Autodesk Inventor part; units mm, degrees
ref_plane "Work Plane1" through (-19.4127, 25.0373, 33.395) normal (0, 0, -1) x (0, 1, 0)
ref_plane "YZ Plane" through (0, 0, 0) normal (1, 0, 0) x (0, 1, 0)
ref_plane "XZ Plane" through (0, 0, 0) normal (0, 1, 0) x (-1, 0, 0)
sketch "Sketch1" plane through (0, 0, 0) normal (0, 0, 1) x (1, 0, 0)
  line L0 (34.925, 95.25) -> (-34.925, 95.25)
  line L1 (-34.925, 95.25) -> (-34.925, 82.55)
  line L2 (-34.925, 82.55) -> (34.925, 82.55)
  line L3 (34.925, 82.55) -> (34.925, 95.25)
  circle A0 centre (-29.0032, 88.9) radius 2.3812
  circle A1 centre (29.0032, 88.9) radius 2.3812
  line L4 (34.925, 6.35) -> (-34.925, 6.35)
  line L5 (-34.925, 6.35) -> (-34.925, -6.35)
  line L6 (-34.925, -6.35) -> (34.925, -6.35)
  line L7 (34.925, -6.35) -> (34.925, 6.35)
  circle A2 centre (-29.0032, 0) radius 2.3812
  circle A3 centre (29.0032, 0) radius 2.3812
  line L8 (34.925, 82.55) -> (34.925, 6.35)
  line L9 (-34.925, 6.35) -> (-34.925, 82.55)
  circle A4 centre (0, 44.45) radius 22.225
  point P0 (0, 0)
  dimension "d0" = 44.45
extrude "Extrusion1" add sketch "Sketch1" along normal blind 12.7
ref_plane "Work Plane1" through (-19.4127, 25.0373, 33.395) normal (0, 0, -1) x (0, 1, 0)
properties part number "Encoder Mount Y"
Verification items for the finished model (mm, model axes). Coordinates: 2 decimals unless noted, no trailing zeros. Order: outer loops, then holes, each group sorted by start corner. A loop starts at its lowest first (then second) coordinate and runs counter-clockwise, first axis right, second up. Notation, with made-up numbers: M -14.5,78.5 L 1.5,78.5 A17 cw 1.5,91.5 Z; hole C -24.5,-25 d2. An arc over 180 degrees is marked long. Return JSON: item names as keys, results as strings.
1) Thickness scan on L1, parallel to Y at x = 0, z = 9.75 (3 decimals); L2, parallel to Y at x = -31, z = 7.75; L3, parallel to Y at x = 30, z = 4. Record the ranges inside material, lowest first. Write a range as [from, to].
Answer list:
{"L1": "[-6.35, 22.225], [66.675, 95.25]", "L2": "[-6.35, -1.3], [1.3, 87.6], [90.2, 95.25]", "L3": "[-6.35, -2.16], [2.16, 86.74], [91.06, 95.25]"}
2) Cross-section at D-D, the plane z = 5.5. Record the boundary of the cut face in (x, y) (3 decimals), and give its area (3 significant figures).
Answer list:
{"outline": "M -34.925,-6.35 L 34.925,-6.35 L 34.925,95.25 L -34.925,95.25 Z; hole C -29.003,0 d4.762; hole C -29.003,88.9 d4.762; hole C 0,44.45 d44.45; hole C 29.003,0 d4.762; hole C 29.003,88.9 d4.762", "area": "5,470 mm2"}
3) Gauge pin test, flat end, axial feed: pin 1 (5.5 mm diameter, centred on x = 29, y = 88.9, fed in from +Z). Record the tip position at first contact, or that the pin passes through.
Answer list:
{"pin 1": "z = 12.7"}
4) Release check for a two-part mould opening along X. For faces 1 (the flat face through (0, 95.25, 6)), 2 (the flat face through (34.925, 44, 6)), 3 (the flat face through (-34.925, 45, 6)), 4 (the cylindrical face through (-31.382, -0.105, 6.261)) record: +X half, -X half, draft (parallel to the pull), parting line (faces both ways), or undercut.
Answer list:
{"face 1": "draft", "face 2": "+X half", "face 3": "-X half", "face 4": "undercut"}
5) Cross-section at B-B, the plane x = 0. Record the boundary of the cut face in (y, z) (3 decimals).
Answer list:
{"outline": "M -6.35,0 L 22.225,0 L 22.225,12.7 L -6.35,12.7 Z; M 66.675,0 L 95.25,0 L 95.25,12.7 L 66.675,12.7 Z"}
6) Cross-section at C-C, the plane y = 88.9. Record the boundary of the cut face in (x, z) (3 decimals), and give its area (3 significant figures).
Answer list:
{"outline": "M -34.925,0 L -31.384,0 L -31.384,12.7 L -34.925,12.7 Z; M -26.622,0 L 26.622,0 L 26.622,12.7 L -26.622,12.7 Z; M 31.384,0 L 34.925,0 L 34.925,12.7 L 31.384,12.7 Z", "area": "766 mm2"}
7) Cross-section at A-A, the plane y = 44.45. Record the boundary of the cut face in (x, z) (3 decimals).
Answer list:
{"outline": "M -34.925,0 L -22.225,0 L -22.225,12.7 L -34.925,12.7 Z; M 22.225,0 L 34.925,0 L 34.925,12.7 L 22.225,12.7 Z"}
